Geometry check sheet. Reference: the model listing, model coordinates, mm. Face numbers are marked on the shaded views. A direction names the side the tool comes from. Coordinates: 2 decimals unless noted, no trailing zeros. Write each loop counter-clockwise with the first axis right and the second up, starting at its lowest first coordinate (ties: lowest second). Pieces come first, ordered by that corner, then holes.
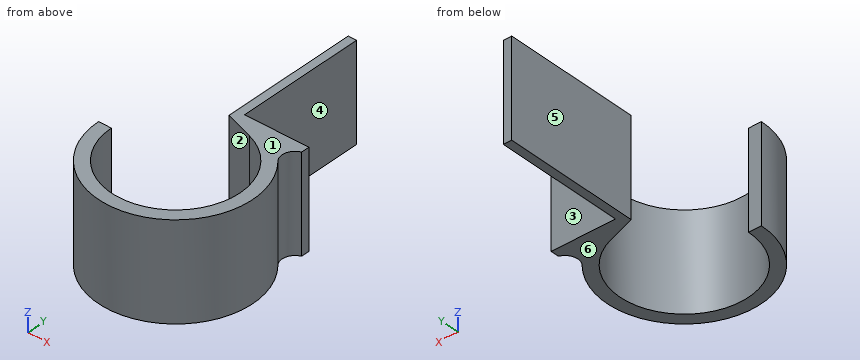
from build123d import *

# Parameters (mm, degrees)
F1_DEPTH    = 19.05
F2_T1_DEPTH = 19.05


# Not quite as in the source:
# - a fillet or chamfer that OpenCascade refuses, or shapes differently, is made with other operations: its cross-section is extruded or revolved along the edge and cut away or added


with BuildPart() as f1:
    # F0 (on Top) → F1 (new body)
    with BuildSketch(Plane.XY):
        Polygon((12.7, 0), (0, 0), (0, -1.651), (6.35, -1.651), (12.7, -1.651), align=None)
        Polygon((0, -1.651), (0, 0), (0, 25.4), (-1.651, 25.4), (-1.651, -1.651), align=None)
        with BuildLine():
            Line((6.35, -1.651), (0, -1.651))
            Line((0, -1.651), (-1.651, -1.651))
            Line((-1.651, -1.651), (4.0781423077, -3.5935831818))
            ThreePointArc((4.0781423077, -3.5935831818), (7.3992429576, -25.9428798508), (-12.7, -15.621))
            Line((-12.7, -15.621), (-15.24, -15.621))
            ThreePointArc((-15.24, -15.621), (7.485390628, -28.8960339791), (7.8868408329, -2.5804731058))
            Line((7.8868408329, -2.5804731058), (6.35, -1.651))
        make_face()
    extrude(amount=F1_DEPTH)

    # F2: fillet of radius 2.54 on 1 edges, made by hand

    # F2_s2 → F2_t1 (join)
    with BuildSketch(Plane.XY):
        with BuildLine():
            ThreePointArc((11.5778863285, -5.7108966623), (11.0593242469, -3.3825527689), (12.7, -1.651))
            Line((12.7, -1.651), (12.619246595, -1.4101787227))
            ThreePointArc((12.619246595, -1.4101787227), (9.525, -1.397), (6.35, -1.397))
            Line((6.35, -1.397), (6.2185526528, -1.8683421149))
            ThreePointArc((6.2185526528, -1.8683421149), (7.7553934856, -2.7978152207), (11.3849215563, -5.8760650512))
            Line((11.3849215563, -5.8760650512), (11.5778863285, -5.7108966623))
        make_face()
    extrude(amount=F2_T1_DEPTH)


solid = f1.part
1. Sectioned sample at C-C, the plane y = 15.5. Record the boundary of the cut face in (x, z), and give its area (3 significant figures).
Computed values:
outline: (-1.65, 0) - (0, 0) - (0, 19.05) - (-1.65, 19.05) - close
area: 31.5 mm2
2. Access from +Z, -Z, +X, -X, +Y, -Y to the whole of each face (thin tool, end or side, straight path). Record for the marked faces 4, 5 and 6.
Computed values:
face 4: +Z, -Z, +X, +Y
face 5: +Z, -Z, -X, +Y
face 6: -Z, +X, -X, +Y, -Y
3. Draft check along Y on the marked faces 1, 2 and 3. Enter one of: released by +Y, released by -Y, zero draft, split by the parting line, or undercut.
Computed values:
face 1: zero draft
face 2: undercut
face 3: released by +Y
4. Thickness scan on line 1 along X through (y, z) = (5.5, 8.25); line 2 along X through (y, z) = (-1, 8.5); line 3 along Y through (x, z) = (6, 16.5). Record the ranges inside material, lowest first.
Computed values:
line 1: x = -1.65 to 0
line 2: x = -1.65 to 12.7
line 3: y = -29.63 to -26.81, -4.43 to 0
5. Sectioned sample at D-D, the plane x = -11.5. Record the boundary of the cut face in (y, z), and give its area (3 significant figures).
Computed values:
outline: (-25.62, 0) - (-21.01, 0) - (-21.01, 19.05) - (-25.62, 19.05) - close
area: 87.8 mm2
6. Sectioned sample at B-B, the plane z = 15.5. Record the boundary of the cut face in (x, y).
Computed values:
outline: (-15.24, -15.62) arc R15.24 ccw (long way) to (11.58, -5.71) arc R2.54 cw to (12.7, -1.65) - (12.7, 0) - (0, 0) - (0, 25.4) - (-1.65, 25.4) - (-1.65, -1.65) - (4.08, -3.59) arc R12.7 cw (long way) to (-12.7, -15.62) - close
7. Gauge pin test, flat ends, axial feed: pin 1 Ø4 at (x, z) = (3, 7) entering from +Y; pin 2 Ø4 at (y, z) = (-20.5, 14) entering from -X; pin 3 Ø4 at (y, z) = (-8, 11) entering from +X. Record the tip position at first contact, or that the pin passes through.
Computed values:
pin 1: stops at y = 0
pin 2: stops at x = -14.97
pin 3: stops at x = 14.17
8. Sectioned sample at A-A, the plane x = 5. Record the boundary of the cut face in (y, z), and give its area (3 significant figures).
Computed values:
outline: (-30.02, 0) - (-27.3, 0) - (-27.3, 19.05) - (-30.02, 19.05) - close; (-3.95, 0) - (0, 0) - (0, 19.05) - (-3.95, 19.05) - close
area: 127 mm2
